Source: CAD feature listing. Evaluate the final solid. Frame: model axes, mm. A direction names the side the tool comes from. Coordinates: 2 decimals unless noted, no trailing zeros. Write each loop counter-clockwise with the first axis right and the second up, starting at its lowest first coordinate (ties: lowest second). Pieces come first, ordered by that corner, then holes. Notation, with made-up numbers: M -18,16 L 27,16 A20 cw 27,40 Z; hole C 39.5,-31.75 d4. An arc over 180 degrees is marked long. Write item = value, one per line. Start each with the question number.
1. Access query for faces 1 (the face through (54, -9, 15)), 2 (the face through (52, -4, 18.75)), 3 (the face through (12, -11, 28)). Directions: +Z, -Z, +X, -X, +Y, -Y. A direction counts if a zero-diameter tool reaches every point of the face in a straight line with its end or side. Return the directions, or none.
2. Section query D-D (y = -10.5). Output: boundary loops of the cut face in (x, z), then the cut area to 3 significant figures.
3. Section query B-B (z = 11.75). Output: boundary loops of the cut face in (x, y), then the cut area to 3 significant figures.
4. Section query C-C (x = 27). Output: boundary loops of the cut face in (y, z).
5. Line query: line 1 along Z through (x, y) = (57.5, -20); line 2 along X through (y, z) = (-13, 12.25); line 3 along X through (y, z) = (-4, 24.25). Output: solid intervals per line, ascending.
6. Section query A-A (y = -3.25). Output: boundary loops of the cut face in (x, z).
7. Pin query (flat end, axial travel): pin 1 Ø8 at (y, z) = (-4.5, 4) entering from -X; pin 2 Ø8 at (x, y) = (32, -17.5) entering from +Z; pin 3 Ø3 at (x, y) = (42, -4) entering from +Z; pin 4 Ø4.5 at (x, y) = (53, -4) entering from +Z. Return the tip coordinate at first contact, or that it passes through.
```python
from build123d import *

# Parameters (mm, degrees)
F0_W     = 61
F0_H     = 22
F1_DEPTH = 28
F3_DEPTH = 22.001
F5_DEPTH = 9


with BuildPart() as f1:
    # F0 (on Top) → F1 (new body)
    with BuildSketch(Plane.XY):
        with Locations((30.5, -11)):
            Rectangle(F0_W, F0_H)
    extrude(amount=F1_DEPTH)

    # F2 (on face) → F3 (cut, through all)
    with BuildSketch(Plane.XZ.offset(22)):
        Polygon((61, 10), (61, 28), (25, 28), align=None)
    extrude(amount=-F3_DEPTH, mode=Mode.SUBTRACT)

    # F4 (on face) → F5 (join)
    with BuildSketch(Plane(origin=(0, 0, 0), x_dir=(-1, 0, 0), z_dir=(0, 1, 0))):
        Polygon((-61, 18.75), (-61, 10), (-43.5, 18.75), align=None)
    extrude(amount=-F5_DEPTH)


solid = f1.part
```
Results are:
q1.face_1 = +Z, +X, -Y
q1.face_2 = +Z, +X, +Y, -Y
q1.face_3 = +Z, +X, -X, +Y, -Y
q2.outline = M 0,0 L 61,0 L 61,10 L 25,28 L 0,28 Z
q2.area = 1,380 mm^2
q3.outline = M 0,-22 L 57.5,-22 L 57.5,-9 L 61,-9 L 61,0 L 0,0 Z
q3.area = 1,300 mm^2
q4.outline = M -22,0 L 0,0 L 0,27 L -22,27 Z
q5.line_1 = 0 to 11.75
q5.line_2 = 0 to 56.5
q5.line_3 = 0 to 32.5
q6.outline = M 0,0 L 61,0 L 61,18.75 L 43.5,18.75 L 25,28 L 0,28 Z
q7.pin_1 = 0
q7.pin_2 = 26.5
q7.pin_3 = 20.25
q7.pin_4 = 18.75
